Verification items for this drawing (mm, ordinates from the low corner). A direction names the side the tool comes from. Give positions to 0.01 mm unless a question says otherwise; leave off trailing zeros. Write each loop counter-clockwise with the first axis right and the second up, starting at its lowest first coordinate (ties: lowest second). Pieces come first, ordered by that corner, then holes. Notation, with made-up numbers: (14, 38.5) -> (28, 38.5) arc R16 cw to (28, 57.5) -> close; hole circle Ø5 at (30, 46). An arc over 180 degrees is marked (long way). Write item = value, one per line.
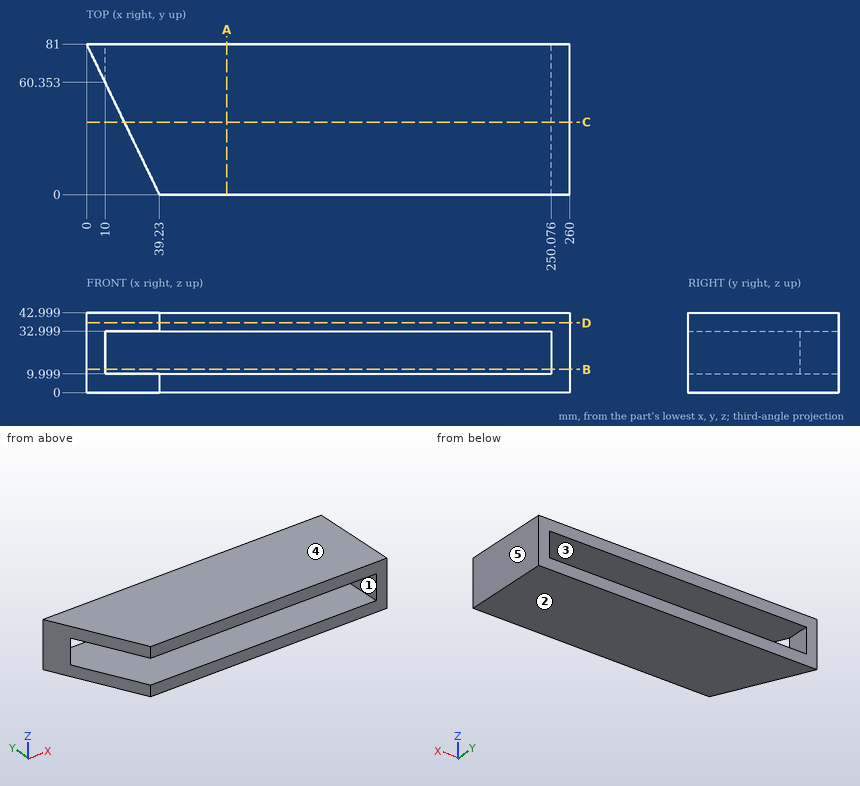
Item 1: Sectioned sample at A-A on x = 75.5. Record the cut outline in (y, z), then the cut area to 3 significant figures.
Response values:
outline = (0, 0) -> (81, 0) -> (81, 10) -> (0, 10) -> close; (0, 33) -> (81, 33) -> (81, 43) -> (0, 43) -> close
area = 1,620 mm^2
Item 2: Go/stop test with flat-tipped pins: P1, Ø12, axis at y = 62.5, z = 27.5, coming from the -X side (1 decimal); P2, Ø7, axis at y = 51.5, z = 16.5, coming from the -X side. Record where each tip stops, or that it passes through.
Response values:
P1 = 6.1
P2 = 250.08
Item 3: Sectioned sample at B-B on z = 12.5. Record the cut outline in (x, y).
Response values:
outline = (0, 81) -> (10, 60.35) -> (10, 81) -> close; (250.08, 0) -> (260, 0) -> (260, 81) -> (250.08, 81) -> close
Item 4: Material ranges on line 1 (Z direction, x = 44.5, y = 36.5); line 2 (X direction, y = 60, z = 15); line 3 (X direction, y = 76.5, z = 20.5) (1 decimal), recorded low to high.
Response values:
line_1 = 0 to 10, 33 to 43
line_2 = 250.08 to 260
line_3 = 2.2 to 10, 250.1 to 260
Item 5: Sectioned sample at D-D on z = 37.5. Record the cut outline in (x, y).
Response values:
outline = (0, 81) -> (39.23, 0) -> (260, 0) -> (260, 81) -> close
Item 6: Sectioned sample at C-C on y = 39. Record the cut outline in (x, z), then the cut area to 3 significant figures.
Response values:
outline = (20.34, 0) -> (260, 0) -> (260, 43) -> (20.34, 43) -> (20.34, 33) -> (250.08, 33) -> (250.08, 10) -> (20.34, 10) -> close
area = 5,020 mm^2
Item 7: Mould release check, pull along X, two halves, no side actions. Record for the marked faces 3, 4 and 5: +X half, -X half, draft (parallel to the pull), parting line (faces both ways), or undercut.
Response values:
face_3 = undercut
face_4 = draft
face_5 = +X half
Item 8: Set-up check for the marked faces 1 and 2: record each of +Z, -Z, +X, -X, +Y, -Y from which the full face is reachable in a straight line by a thin tool's end or side.
Response values:
face_1 = +Y, -Y
face_2 = -Z, +X, -X, +Y, -Y
